For this review, take the finished solid that the model builds, in its own axes (mm). A direction names the side the tool comes from. Give positions to 0.01 mm unless a question says otherwise; leave off trailing zeros. Write each loop counter-clockwise with the first axis right and the second up, starting at its lowest first coordinate (ties: lowest second). Pieces come first, ordered by that corner, then holes.
from build123d import *

# Parameters (mm, degrees)
SKETCH_1_W          = 30
SKETCH_1_H          = 30
EXTRUDE_1_DEPTH     = 30
SKETCH_2_R          = 7.5
EXTRUDE_2_DEPTH     = 220
SKETCH_3_R          = 7.5
EXTRUDE_3_DEPTH     = 50
SKETCH_4_W          = 30
SKETCH_4_H          = 30
EXTRUDE_4_DEPTH     = 30
SKETCH_5_R          = 4
CUT_EXTRUDE_1_DEPTH = 31


with BuildPart() as part:
    # 草图1 → 凸台-拉伸1 (new body)
    with BuildSketch(Plane.XY):
        Rectangle(SKETCH_1_W, SKETCH_1_H)
    extrude(amount=EXTRUDE_1_DEPTH)

    # 草图2 → 凸台-拉伸2 (add)
    with BuildSketch(Plane(origin=(0, 0, 0), x_dir=(-1, 0, 0), z_dir=(0, 0, -1))):
        Circle(SKETCH_2_R)
    extrude(amount=EXTRUDE_2_DEPTH)

    # 草图3 → 凸台-拉伸3 (add)
    with BuildSketch(Plane.XZ.offset(15)):
        with Locations((0, 15)):
            Circle(SKETCH_3_R)
    extrude_3 = extrude(amount=EXTRUDE_3_DEPTH)

    # 草图4 → 凸台-拉伸4 (add)
    with BuildSketch(Plane.XZ.offset(65)):
        with Locations((0, 15)):
            Rectangle(SKETCH_4_W, SKETCH_4_H)
    extrude_4 = extrude(amount=EXTRUDE_4_DEPTH)

    # 草图5 → 切除-拉伸1 (cut, through all)
    with BuildSketch(Plane.ZY.offset(15)):
        with Locations((15, -80)):
            Circle(SKETCH_5_R)
    cut_extrude_1 = extrude(amount=-CUT_EXTRUDE_1_DEPTH, mode=Mode.SUBTRACT)

    # 镜向1: 凸台-拉伸3, 凸台-拉伸4, 切除-拉伸1 across plane
    add(extrude_3.mirror(Plane.ZX))
    add(extrude_4.mirror(Plane.ZX))
    add(cut_extrude_1.mirror(Plane.ZX), mode=Mode.SUBTRACT)


solid = part.part
(1) Tool access review of faces 4 (the flat face through (0, -80, 0)), 5 (the cylindrical face through (-5.5, -39.6, 20.1)), 6 (the flat face through (0, 80, 0)): name each direction out of +Z, -Z, +X, -X, +Y, -Y from which nothing blocks a thin tool from reaching the whole face with its end or side.
(2) We need section B-B (y = 80). Write out the cut boundary in (x, z), and give its area (3 significant figures).
(3) We need section D-D (x = 0). Write out the cut boundary in (y, z), and give its area (3 significant figures).
(4) The part is to be moulded in two halves that separate along Z. For faces 1 (the cylindrical face through (-0.21, 83.905, 14.133)), 2 (the cylindrical face through (7.493, 0.33, -108.46)), 3 (the flat face through (-4, 7, 0)), say which applies: +Z half, -Z half, draft (parallel to the pull), parting line (faces both ways), or undercut.
(5) We need section C-C (y = 0). Write out the cut boundary in (x, z).
(6) For L1, parallel to Y at x = 3, z = 15; L2, parallel to Y at x = -7.75, z = 15; L3, parallel to Z at x = -1, y = 80, list the stretches that pass through material, from the lowest coordinate up.
(7) Clearance check with flat-ended pins moving along their axes: pin 1 Ø2 at (x, z) = (-0.5, -84) entering from -Y; pin 2 Ø15 at (x, y) = (2.5, -78) entering from -Z; pin 3 Ø5 at (x, z) = (7.5, -139.5) entering from -Y; pin 4 Ø7 at (y, z) = (-80, 15) entering from -X. State where each tip first meets the part, or that it passes through.
(8) We need section A-A (z = 15). Write out the cut boundary in (x, y), and give its area (3 significant figures).
The answers:
1. face 4: -Z, +X, -X, -Y
1. face 5: none
1. face 6: -Z, +X, -X, +Y
2. outline: (-15, 0) - (15, 0) - (15, 11) - (-15, 11) - close; (-15, 19) - (15, 19) - (15, 30) - (-15, 30) - close
2. area: 660 mm2
3. outline: (-95, 0) - (-65, 0) - (-65, 7.5) - (-15, 7.5) - (-15, 0) - (-7.5, 0) - (-7.5, -220) - (7.5, -220) - (7.5, 0) - (15, 0) - (15, 7.5) - (65, 7.5) - (65, 0) - (95, 0) - (95, 30) - (65, 30) - (65, 22.5) - (15, 22.5) - (15, 30) - (-15, 30) - (-15, 22.5) - (-65, 22.5) - (-65, 30) - (-95, 30) - close; hole circle Ø8 at (-80, 15); hole circle Ø8 at (80, 15)
3. area: 7,400 mm2
4. face 1: undercut
4. face 2: draft
4. face 3: -Z half
5. outline: (-15, 0) - (-7.5, 0) - (-7.5, -220) - (7.5, -220) - (7.5, 0) - (15, 0) - (15, 30) - (-15, 30) - close
6. L1: y = -95 to -84, -76 to 76, 84 to 95
6. L2: y = -95 to -84, -76 to -65, -15 to 15, 65 to 76, 84 to 95
6. L3: z = 0 to 11, 19 to 30
7. pin 1: stops at y = -7.5
7. pin 2: stops at z = 0
7. pin 3: stops at y = -5.59
7. pin 4: passes through
8. outline: (-15, -95) - (15, -95) - (15, -84) - (-15, -84) - close; (-15, -76) - (15, -76) - (15, -65) - (7.5, -65) - (7.5, -15) - (15, -15) - (15, 15) - (7.5, 15) - (7.5, 65) - (15, 65) - (15, 76) - (-15, 76) - (-15, 65) - (-7.5, 65) - (-7.5, 15) - (-15, 15) - (-15, -15) - (-7.5, -15) - (-7.5, -65) - (-15, -65) - close; (-15, 84) - (15, 84) - (15, 95) - (-15, 95) - close
8. area: 3,720 mm2
